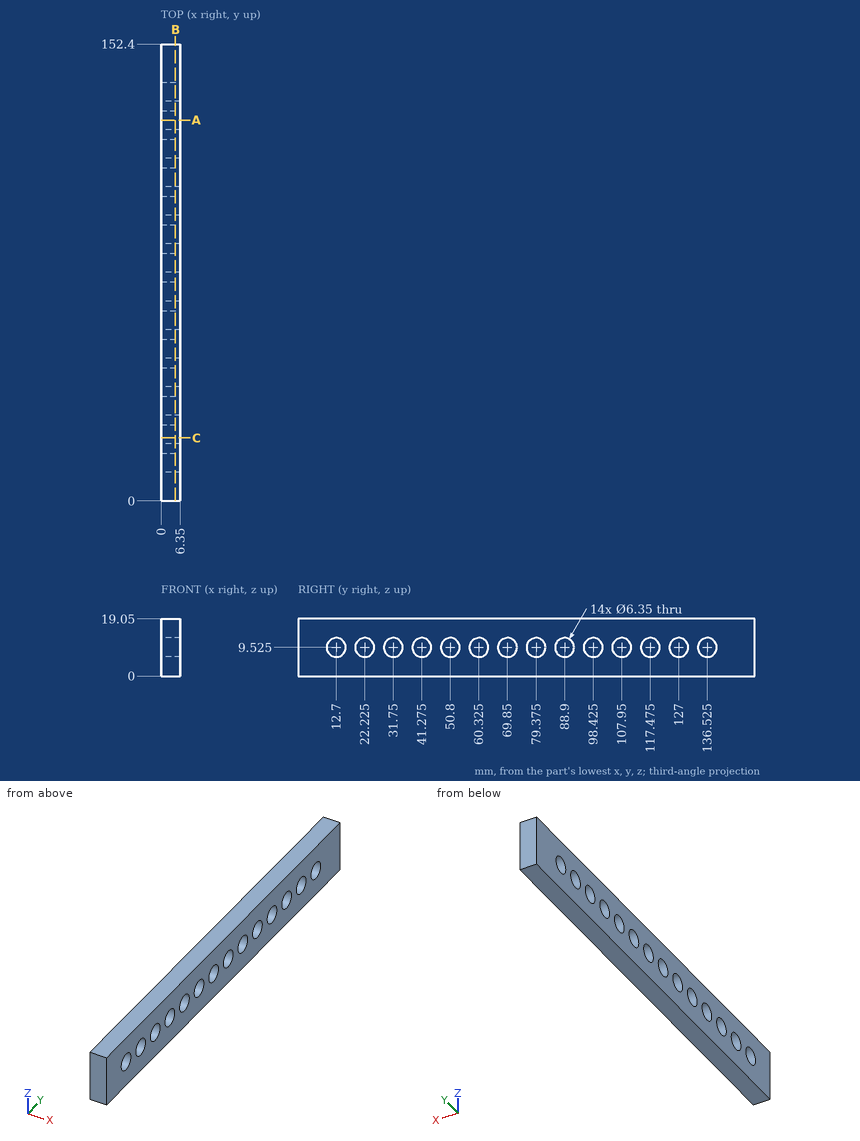
Input: dimensioned drawing with shaded views. Units: mm. Origin: part minimum x, y, z. Coordinates: 2 decimals unless noted, no trailing zeros. Write each loop counter-clockwise with the first axis right and the second up, starting at its lowest first coordinate (ties: lowest second). Pieces come first, ordered by that corner, then holes. Notation, with made-up numbers: M -25,36 L -9,36 A31 ccw -9,75 Z; hole C 63,-3 d7. An arc over 180 degrees is marked long. Answer as CSV lines item,"result". Start each with the question number.
Q1. Cut plane C-C on y = 21. Return the cut outline in (x, z), then the cut area to 3 significant figures.
Q2. Cut plane A-A on y = 127. Return the cut outline in (x, z).
Q3. Line query: line 1 (Z direction, x = 5, y = 22.5); line 2 (Z direction, x = 3, y = 78.5). Output: solid intervals per line, ascending. Write a range as from..to.
Q4. Cut plane B-B on x = 4.75. Count the separate pieces of the cut face and the enclosed holes in it, then the cut area to 3 significant figures.
Findings below:
1,outline,"M 0,0 L 6.35,0 L 6.35,6.6 L 0,6.6 Z; M 0,12.45 L 6.35,12.45 L 6.35,19.05 L 0,19.05 Z"
1,area,"83.8 mm2"
2,outline,"M 0,0 L 6.35,0 L 6.35,6.35 L 0,6.35 Z; M 0,12.7 L 6.35,12.7 L 6.35,19.05 L 0,19.05 Z"
3,line 1,"z = 0..6.36, 12.69..19.05"
3,line 2,"z = 0..6.47, 12.58..19.05"
4,separate pieces,"1"
4,enclosed holes,"14"
4,area,"2,460 mm2"
